Check sheet for the modelled part. Datum: model origin and axes. Units: mm. A direction names the side the tool comes from. Give positions to 0.01 mm unless a question says otherwise; leave off trailing zeros. Loops run counter-clockwise (first coordinate to the right, second up) from the corner with the lowest first, then second, coordinate; pieces in that order, holes last. Notation, with made-up numbers: M 7.5,52 L 58.5,52 A14 cw 58.5,72 Z; hole C 6,20.25 d3. An arc over 180 degrees is marked long. Use one line per item in the form item = value.
Autodesk Inventor part; units mm, degrees
ref_plane "YZ Plane" through (0, 0, 0) normal (1, 0, 0) x (0, 1, 0)
ref_plane "XZ Plane" through (0, 0, 0) normal (0, 1, 0) x (-1, 0, 0)
ref_plane "XY Plane" through (0, 0, 0) normal (0, 0, 1) x (1, 0, 0)
sketch "Skizze1" plane through (0, 0, 0) normal (1, 0, 0) x (0, 1, 0)
  line L0 (-12.5, 30) -> (12.5, 30)
  line L1 (12.5, 30) -> (12.5, -30)
  line L2 (12.5, -30) -> (-12.5, -30)
  line L3 (-12.5, -30) -> (-12.5, 30)
  line L4 (-12.5, 30) -> (12.5, -30) construction
  line L5 (12.5, 30) -> (-12.5, -30) construction
  point P0 (0, 0)
  dimension "d0" = 25
  dimension "d1" = 60
extrude "Extrusion1" add sketch "Skizze1" along normal blind 32.5
sketch "Skizze2" plane through (32.5, 0, 0) normal (1, 0, 0) x (0, 0, -1)
  line L0 (-30, -12.5) -> (30, -12.5) construction
  line L1 (0, -12.5) -> (17, -12.5) construction
  line L2 (17, -12.5) -> (-17, -12.5)
  line L3 (-17, -12.5) -> (-17, 21.5)
  line L4 (-17, 21.5) -> (17, 21.5)
  line L5 (17, 21.5) -> (17, -12.5)
  point P0 (0, 0)
  dimension "d4" = 17
  dimension "d5" = 34
  dimension "d6" = 34
extrude "Extrusion2" add sketch "Skizze2" along normal blind 10.5
extrude "Extrusion3" add sketch "Skizze2" against normal blind 23.5
sketch "Skizze3" plane through (43, 21.5, 17) normal (0, 1, 0) x (1, 0, 0)
  line L0 (-34, 0) -> (-34, 34) construction
  line L1 (-10.5, 34) -> (0, 34) construction
  line L2 (-34, 0) -> (0, 34) construction
  line L3 (0, 34) -> (0, 0) construction
  line L4 (-34, 34) -> (0, 0) construction
  point P0 (-43, 17)
sketch "Skizze4" plane through (43, 21.5, 17) normal (0, 1, 0) x (1, 0, 0)
  point P0 (-43, 17)
  point P1 (-17, 17)
hole "Bohrung1" at (26, 21.5, 0) direction (0, -1, 0) diameter 16 end through all
sketch "Skizze5" plane through (32.5, 0, 0) normal (1, 0, 0) x (0, 0, -1)
  line L0 (-17, 21.5) -> (-17, -12.5) construction
  line L1 (-17, 12.5) -> (-30, 12.5) construction
  line L2 (-30, 12.5) -> (-30, -12.5) construction
  line L3 (-30, -12.5) -> (-17, -12.5) construction
  line L4 (-30, 12.5) -> (30, 12.5) construction
  line L5 (-23.5, 12.5) -> (-23.5, -12.5) construction
  line L6 (30, -12.5) -> (-30, -12.5) construction
  line L7 (-23.5, 12.5) -> (-23.5, 6.5) construction
  line L8 (-23.5, 6.5) -> (-23.5, -6.5) construction
  line L9 (-23.5, 6.5) -> (22.5, 6.5) construction
  line L10 (22.5, 6.5) -> (22.5, -6.5) construction
  point P0 (0, 0)
  dimension "d18" = 6
  dimension "d19" = 13
  dimension "d20" = 46
  dimension "d21" = 13
hole "Bohrung2" at (32.5, 6.5, 23.5) at (32.5, -6.5, 23.5) at (32.5, 6.5, -22.5) at (32.5, -6.5, -22.5) direction (-1, 0, 0) diameter 6.6 end through all counterbore diameter 11 counterbore depth 6
properties part number "Festlager" material "Eisen, Grau"
1) Section check B-B (x = 7). Record the cut outline in (y, z), then the cut area to 3 significant figures.
Evaluation:
outline = M -12.5,-30 L 12.5,-30 L 12.5,30 L -12.5,30 Z; hole C -6.5,-22.5 d6.6; hole C -6.5,23.5 d6.6; hole C 6.5,-22.5 d6.6; hole C 6.5,23.5 d6.6
area = 1,360 mm^2
2) Section check A-A (z = 23.5). Record the cut outline in (x, y).
Evaluation:
outline = M 0,-12.5 L 32.5,-12.5 L 32.5,-12 L 26.5,-12 L 26.5,-9.8 L 0,-9.8 Z; M 0,-3.2 L 26.5,-3.2 L 26.5,-1 L 32.5,-1 L 32.5,1 L 26.5,1 L 26.5,3.2 L 0,3.2 Z; M 0,9.8 L 26.5,9.8 L 26.5,12 L 32.5,12 L 32.5,12.5 L 0,12.5 Z
3) Section check C-C (z = 0). Record the cut outline in (x, y), then the cut area to 3 significant figures.
Evaluation:
outline = M 0,-12.5 L 18,-12.5 L 18,21.5 L 9,21.5 L 9,12.5 L 0,12.5 Z; M 34,-12.5 L 43,-12.5 L 43,21.5 L 34,21.5 Z
area = 837 mm^2
4) Section check D-D (y = 5). Record the cut outline in (x, z), then the cut area to 3 significant figures.
Evaluation:
outline = M 0,-30 L 32.5,-30 L 32.5,-27.79 L 26.5,-27.79 L 26.5,-25.44 L 0,-25.44 Z; M 0,-19.56 L 26.5,-19.56 L 26.5,-17.21 L 32.5,-17.21 L 32.5,-17 L 43,-17 L 43,17 L 32.5,17 L 32.5,18.21 L 26.5,18.21 L 26.5,20.56 L 0,20.56 Z; M 0,26.44 L 26.5,26.44 L 26.5,28.79 L 32.5,28.79 L 32.5,30 L 0,30 Z; hole C 26,0 d16
area = 1,670 mm^2
5) Set-up check for faces 1 (the face through (33, 9, -17)), 2 (the face through (33, 8, 17)), 3 (the face through (29.46, 8.61, 18.42)): record each of +Z, -Z, +X, -X, +Y, -Y from which the full face is reachable in a straight line by a thin tool's end or side.
Evaluation:
face_1 = -Z, +X, +Y
face_2 = +Z, +X, +Y
face_3 = +X
6) Release check for a two-part mould opening along Y. For faces 4 (the face through (9, 17, 0)), 5 (the face through (22, 21.5, -7.3)), 6 (the face through (26.5, 9, 21)) record: pulls with the +Y half, pulls with the -Y half, needs draft (parallel to the pull), parting line crosses it, or undercut.
Evaluation:
face_4 = needs draft
face_5 = pulls with the +Y half
face_6 = undercut
7) Depth check by flat-ended pin: pin 1 Ø4 at (x, y) = (10, 16) entering from -Z; pin 2 Ø10 at (y, z) = (6.5, -22.5) entering from +X; pin 3 Ø8 at (x, z) = (30.5, 23) entering from +Y. Enter the tip coordinate at first touch or a pass-through.
Evaluation:
pin_1 = -17
pin_2 = 26.5
pin_3 = 12.5
8) Scan lines: line 1 (Y direction, x = 28.15, z = 23.5); line 2 (Z direction, x = 14, y = -6.5); line 3 (Y direction, x = 13, z = -22). Record each from-to range of solid material in increasing order.
Evaluation:
line_1 = -12.5 to -12, -1 to 1, 12 to 12.5
line_2 = -30 to -25.8, -19.2 to 20.2, 26.8 to 30
line_3 = -12.5 to -9.76, -3.24 to 3.24, 9.76 to 12.5
